from build123d import *

# Parameters (mm, degrees)
F0_W     = 160
F0_H     = 100
F1_DEPTH = 30
F3_DEPTH = 25
F5_DEPTH = 25
F6_R     = 5
F7_R     = 5
F8_R     = 5


with BuildPart() as f1:
    # F0 (on Top) → F1 (new body)
    with BuildSketch(Plane.XY):
        Rectangle(F0_W, F0_H)
    extrude(amount=F1_DEPTH)

    # F2 (on face) → F3 (cut)
    with BuildSketch(Plane.XY.offset(30)):
        Polygon((-70.5, -48), (-55.5, -48), (-48, -35.009619), (-55.5, -22.019238), (-70.5, -22.019238), (-78, -35.009619), align=None)
        Polygon((-31.267949, -8.028857), (-46.267949, -8.028857), (-53.767949, -21.019238), (-46.267949, -34.009619), (-31.267949, -34.009619), (-23.767949, -21.019238), align=None)
        Polygon((-7.035898, 5.961524), (-22.035898, 5.961524), (-29.535898, -7.028857), (-22.035898, -20.019238), (-7.035898, -20.019238), (0.464102, -7.028857), align=None)
        Polygon((17.196152, 19.951905), (2.196152, 19.951905), (-5.303848, 6.961524), (2.196152, -6.028857), (17.196152, -6.028857), (24.696152, 6.961524), align=None)
        Polygon((41.428203, 33.942286), (26.428203, 33.942286), (18.928203, 20.951905), (26.428203, 7.961524), (41.428203, 7.961524), (48.928203, 20.951905), align=None)
        Polygon((-7.035898, -22.019238), (-22.035898, -22.019238), (-29.535898, -35.009619), (-22.035898, -48), (-7.035898, -48), (0.464102, -35.009619), align=None)
        Polygon((17.196152, -8.028857), (2.196152, -8.028857), (-5.303848, -21.019238), (2.196152, -34.009619), (17.196152, -34.009619), (24.696152, -21.019238), align=None)
        Polygon((41.428203, 5.961524), (26.428203, 5.961524), (18.928203, -7.028857), (26.428203, -20.019238), (41.428203, -20.019238), (48.928203, -7.028857), align=None)
        Polygon((65.660254, 19.951905), (50.660254, 19.951905), (43.160254, 6.961524), (50.660254, -6.028857), (65.660254, -6.028857), (73.160254, 6.961524), align=None)
        Polygon((41.428203, -22.019238), (26.428203, -22.019238), (18.928203, -35.009619), (26.428203, -48), (41.428203, -48), (48.928203, -35.009619), align=None)
        Polygon((65.660254, -8.028857), (50.660254, -8.028857), (43.160254, -21.019238), (50.660254, -34.009619), (65.660254, -34.009619), (73.160254, -21.019238), align=None)
    extrude(amount=-F3_DEPTH, mode=Mode.SUBTRACT)

    # F4 (on face) → F5 (cut, through all)
    with BuildSketch(Plane.XY.offset(30)):
        Polygon((51.196152, 21.951905), (78, 21.951905), (78, 48), (42.549597, 48), (42.549597, 35.999976), (50.392305, 22.416007), align=None)
        Polygon((16.891695, 22.092275), (17.743567, 22.433024), (25.18436, 35.821269), (25.18436, 48), (-78, 48), (-78, -31.009619), (-71.654701, -20.019238), (-55.989621, -20.019238), (-55.132385, -19.572759), (-47.427833, -6.022478), (-31.684874, -6.108645), (-30.913347, -5.594294), (-23.198907, 7.961524), (-7.571797, 7.961524), (-6.767949, 8.425626), (1.035106, 21.940913), align=None)
        Polygon((40.549597, 48.023537), (27.18436, 48.023537), (27.18436, 35.942286), (33.928203, 35.942286), (40.549597, 35.942286), align=None)
    extrude(amount=-F5_DEPTH, mode=Mode.SUBTRACT)

    # F6
    f6_edges = [f1.edges().sort_by_distance(p)[0] for p in [
        (-46.267949, -8.028857, 17.5),
        (-31.267949, -8.028857, 17.5),
    ]]
    fillet(f6_edges, radius=F6_R)

    # F7
    f7_edges = [f1.edges().sort_by_distance(p)[0] for p in [
        (-80, -50, 15),
        (80, -50, 15),
        (80, 50, 15),
        (-80, 50, 15),
        (-78, 48, 17.5),
        (78, 48, 17.5),
    ]]
    fillet(f7_edges, radius=F7_R)

    # F8
    f8_edges = [f1.edges().sort_by_distance(p)[0] for p in [
        (-23.198907, 7.961524, 17.5),
        (1.035106, 21.940913, 17.5),
        (-47.427833, -6.022478, 17.5),
        (-71.654701, -20.019238, 17.5),
        (-70.5, -22.019238, 17.5),
        (-22.035898, 5.961524, 17.5),
        (2.196152, 19.951905, 17.5),
    ]]
    fillet(f8_edges, radius=F8_R)


solid = f1.part
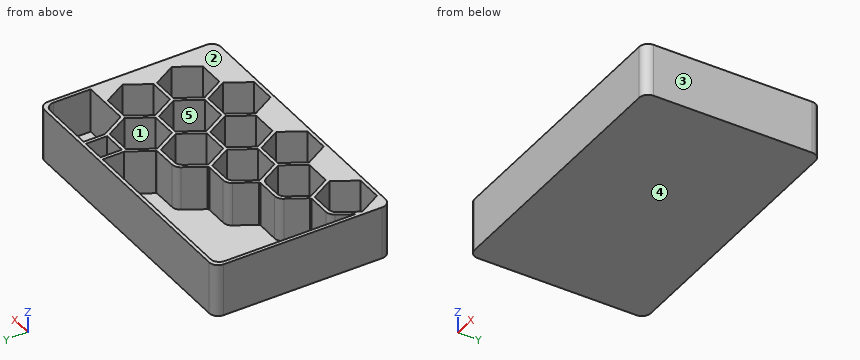
Source: CAD feature listing. Evaluate the final solid. Frame: model axes, mm. Face numbers are marked on the shaded views. A direction names the side the tool comes from. Round coordinates to 2 decimals unless told otherwise and drop trailing zeros. Write each loop counter-clockwise with the first axis right and the second up, starting at its lowest first coordinate (ties: lowest second). Pieces come first, ordered by that corner, then holes. Notation, with made-up numbers: M 17,-24.75 L 49,-24.75 A13 cw 49,-3.75 Z; hole C 53,-39 d8. An arc over 180 degrees is marked long. One line per item, written item: value. Start each with the question number.
Item 1: Section query C-C (y = 11). Return the cut outline in (x, z), plus the area to 3 significant figures.
Item 2: Section query B-B (z = 15). State how many separate pieces and enclosed holes the cut face has, plus the area to 3 significant figures.
Item 3: Ray query, L1, parallel to Y at x = 56.5, z = 6.75; L2, parallel to X at y = 41, z = 12.5; L3, parallel to Y at x = -66, z = 18.25. Return the intervals inside material, ascending. Write a range as from..to.
Item 4: Section query A-A (x = -12). Return the cut outline in (y, z).
Item 5: Section query D-D (x = -62). Return the cut outline in (y, z).
Item 6: Set-up query: the marked faces 4 and 5. Return all of +Z, -Z, +X, -X, +Y, -Y with unobstructed straight access to the full face (end or side cutting, diameter ignored); none if empty.
Item 7: Pin query (flat end, axial travel): pin 1 (5 mm diameter, centred on x = 63, y = -26, fed in from +Z). Return the tip coordinate at first contact, or that it passes through.
Item 8: Mould query, pull axis X, two halves, no side actions, for the marked faces 1, 2 and 3. Classes: pulls with the +X half, pulls with the -X half, needs draft (parallel to the pull), parting line crosses it, or undercut.
Result set:
1. outline: M -80,0 L 80,0 L 80,30 L 70.83,30 L 70.83,5 L 45.49,5 L 45.49,30 L 43.18,30 L 43.18,5 L 24.67,5 L 24.67,30 L 22.36,30 L 22.36,5 L -2.97,5 L -2.97,30 L -5.28,30 L -5.28,5 L -78,5 L -78,30 L -80,30 Z
1. area: 1,250 mm²
2. separate pieces: 1
2. enclosed holes: 14
2. area: 3,730 mm²
3. L1: y = -50..-34.01, -8.03..-6.03, 19.95..21.95, 48..50
3. L2: x = -80..-78, 25.18..27.18, 40.55..42.55, 78..80
3. L3: y = -50..-48, -22.02..-20.02, 48..50
4. outline: M -50,0 L 50,0 L 50,30 L 48,30 L 48,5 L 7.96,5 L 7.96,30 L 5.96,30 L 5.96,5 L -20.02,5 L -20.02,30 L -22.02,30 L -22.02,5 L -48,5 L -48,30 L -50,30 Z
5. outline: M -50,0 L 50,0 L 50,30 L 48,30 L 48,5 L -20.02,5 L -20.02,30 L -22.02,30 L -22.02,5 L -48,5 L -48,30 L -50,30 Z
6. face 4: -Z, +X, -X, +Y, -Y
6. face 5: +Z
7. pin 1: stops at z = 5
8. face 1: undercut
8. face 2: needs draft
8. face 3: pulls with the +X half
